```python
from build123d import *

# Parameters (mm, degrees)
EXTRUDE_1_DEPTH            = 4
SKETCH_4_W                 = 1.5
SKETCH_4_H                 = 8
SKETCH_4_W_2               = 8
SKETCH_4_H_2               = 1.5
EXTRUDE_2_DEPTH            = 1
MIRROR_2_COPY_1_DEPTH      = 4
MIRROR_2_COPY_3_SKETCH_W   = 1.5
MIRROR_2_COPY_3_SKETCH_H   = 8
MIRROR_2_COPY_3_SKETCH_W_2 = 8
MIRROR_2_COPY_3_SKETCH_H_2 = 1.5
MIRROR_2_COPY_3_DEPTH      = 1


with BuildPart() as part:
    # Эскиз1 → Бобышка-Вытянуть1 (new body)
    with BuildSketch(Plane.XY):
        with BuildLine():
            Line((0, 0), (0, 28))
            Line((0, 28), (4, 28))
            ThreePointArc((4, 28), (20.970562748, 20.970562748), (28, 4))
            Line((28, 4), (28, 0))
            Line((28, 0), (0, 0))
        make_face()
    extrude_1 = extrude(amount=EXTRUDE_1_DEPTH)

    # Эскиз3 → Зенковка для винта с полупотайной головкой M81 (revolve, cut)
    with BuildSketch(Plane(origin=(14, 14, 4), x_dir=(0, -1, 0), z_dir=(1, 0, 0))):
        Polygon((0, 0), (0, 11.953872786), (4.5, 9.25), (4.5, 3.5), (8, 0), align=None)
    hole_wizard_m81 = revolve(axis=Axis((14, 14, 10.35), (0, 0, -1)), mode=Mode.SUBTRACT)

    # Эскиз4 → Бобышка-Вытянуть2 (add)
    with BuildSketch(Plane(origin=(0, 0, 0), x_dir=(-1, 0, 0), z_dir=(0, 0, -1))):
        with Locations((-2.25, 14)):
            Rectangle(SKETCH_4_W, SKETCH_4_H)
        with Locations((-14, 2.25)):
            Rectangle(SKETCH_4_W_2, SKETCH_4_H_2)
    extrude_2 = extrude(amount=EXTRUDE_2_DEPTH)

    # Зеркальное отражение1: Бобышка-Вытянуть1, Зенковка для винта с полупотайной головкой M81, Бобышка-Вытянуть2 across plane
    add(extrude_1.mirror(Plane(origin=(0, 0, 0), x_dir=(0, 0.707106781, 0.707106781), z_dir=(0, -0.707106781, 0.707106781))))
    add(hole_wizard_m81.mirror(Plane(origin=(0, 0, 0), x_dir=(0, 0.707106781, 0.707106781), z_dir=(0, -0.707106781, 0.707106781))), mode=Mode.SUBTRACT)
    add(extrude_2.mirror(Plane(origin=(0, 0, 0), x_dir=(0, 0.707106781, 0.707106781), z_dir=(0, -0.707106781, 0.707106781))))

    # Зеркальное отражение2: Бобышка-Вытянуть1, Зенковка для винта с полупотайной головкой M81, Бобышка-Вытянуть2 across plane
    add(extrude_1.mirror(Plane(origin=(0, 0, 0), x_dir=(0.707106781, 0, 0.707106781), z_dir=(-0.707106781, 0, 0.707106781))))
    add(hole_wizard_m81.mirror(Plane(origin=(0, 0, 0), x_dir=(0.707106781, 0, 0.707106781), z_dir=(-0.707106781, 0, 0.707106781))), mode=Mode.SUBTRACT)
    add(extrude_2.mirror(Plane(origin=(0, 0, 0), x_dir=(0.707106781, 0, 0.707106781), z_dir=(-0.707106781, 0, 0.707106781))))

    # Зеркальное отражение2 copy 1 sketch → Зеркальное отражение2 copy 1 (add)
    with BuildSketch(Plane.ZX):
        with BuildLine():
            Line((0, 0), (0, 28))
            Line((0, 28), (4, 28))
            ThreePointArc((4, 28), (20.970562748, 20.970562748), (28, 4))
            Line((28, 4), (28, 0))
            Line((28, 0), (0, 0))
        make_face()
    extrude(amount=MIRROR_2_COPY_1_DEPTH)

    # Зеркальное отражение2 copy 2 sketch → Зеркальное отражение2 copy 2 (revolve, cut)
    with BuildSketch(Plane(origin=(14, 4, 14), x_dir=(-1, 0, 0), z_dir=(0, 0, 1))):
        Polygon((0, 0), (0, 11.953872786), (4.5, 9.25), (4.5, 3.5), (8, 0), align=None)
    revolve(axis=Axis((14, 10.35, 14), (0, -1, 0)), mode=Mode.SUBTRACT)

    # Зеркальное отражение2 copy 3 sketch → Зеркальное отражение2 copy 3 (add)
    with BuildSketch(Plane(origin=(0, 0, 0), x_dir=(0, 0, -1), z_dir=(0, -1, 0))):
        with Locations((-2.25, 14)):
            Rectangle(MIRROR_2_COPY_3_SKETCH_W, MIRROR_2_COPY_3_SKETCH_H)
        with Locations((-14, 2.25)):
            Rectangle(MIRROR_2_COPY_3_SKETCH_W_2, MIRROR_2_COPY_3_SKETCH_H_2)
    extrude(amount=MIRROR_2_COPY_3_DEPTH)


solid = part.part
```
Check sheet for the modelled part. Datum: model origin and axes. Units: mm. A direction names the side the tool comes from. Coordinates: 2 decimals unless noted, no trailing zeros. Order: outer loops, then holes, each group sorted by start corner. A loop starts at its lowest first (then second) coordinate and runs counter-clockwise, first axis right, second up. Notation, with made-up numbers: (87.5, -23.5) -> (146.5, -23.5) arc R17 ccw to (146.5, -17.5) -> close; hole circle Ø8 at (-34.75, 34). An arc over 180 degrees is marked (long way). Write each question's results on one line, items separated by ' | '. Start each with the question number.
1) Depth check by flat-ended pin: pin 1 (0.5 mm diameter, centred on x = -0.5, y = 15, fed in from +Z); pin 2 (3 mm diameter, centred on x = 15.5, z = 21, fed in from -Y); pin 3 (10 mm diameter, centred on y = 10.5, z = 23.5, fed in from -X); pin 4 (1.5 mm diameter, centred on x = 3.5, z = 13.5, fed in from -Y). Enter the tip coordinate at first touch or a pass-through.
2) Section check A-A (z = 1). Enter the section's corners in (x, y).
3) Section check B-B (z = 14). Enter the section's corners in (x, y), and give its area (3 significant figures).
4) Material ranges on line 1 along Y through (x, z) = (12, 26.25); line 2 along Y through (x, z) = (4, 0.75); line 3 along Z through (x, y) = (3.5, 10.75), recorded low to high.
5) Draft check along X on faces 1 (the face through (2, 2, 28)), 2 (the face through (9.54, 14.59, 0.25)), 3 (the face through (3, 13.9, -0.5)). Enter one of: pulls with the +X half, pulls with the -X half, needs draft (parallel to the pull), parting line crosses it, or undercut.
6) Section check D-D (x = 26.25). Enter the section's corners in (y, z), and give its area (3 significant figures).
7) Set-up check for faces 4 (the face through (14.1, -0.5, 3)), 5 (the face through (14.1, 3, -0.5)), 6 (the face through (3, -0.5, 13.9)): record each of +Z, -Z, +X, -X, +Y, -Y from which the full face is reachable in a straight line by a thin tool's end or side.
Checked values:
1) pin 1: z = 3 | pin 2: y = 0 | pin 3: x = 0 | pin 4: y = -1
2) outline: (0, 0) -> (28, 0) -> (28, 4) arc R24 ccw to (4, 28) -> (0, 28) -> close; hole circle Ø10 at (14, 14)
3) outline: (-1, 1.5) -> (0, 1.5) -> (0, 0) -> (1.5, 0) -> (1.5, -1) -> (3, -1) -> (3, 0) -> (9.5, 0) -> (9.5, 0.5) -> (6, 4) -> (4, 4) -> (4, 6) -> (0.5, 9.5) -> (0, 9.5) -> (0, 3) -> (-1, 3) -> close; (0, 18.5) -> (0.5, 18.5) -> (4, 22) -> (4, 25.82) -> (0, 25.82) -> close; (18.5, 0) -> (25.82, 0) -> (25.82, 4) -> (22, 4) -> (18.5, 0.5) -> close | area: 97.0 mm²
4) line 1: 0 to 4 | line 2: 0 to 28 | line 3: 0 to 7.24, 20.76 to 27.03
5) face 1: needs draft | face 2: undercut | face 3: pulls with the +X half
6) outline: (0, 0) -> (13, 0) -> (13, 4) -> (4, 4) -> (4, 13) -> (0, 13) -> close | area: 88.0 mm²
7) face 4: +Z, +X, -X, -Y | face 5: -Z, +X, -X, +Y | face 6: +Z, -Z, +X, -Y
